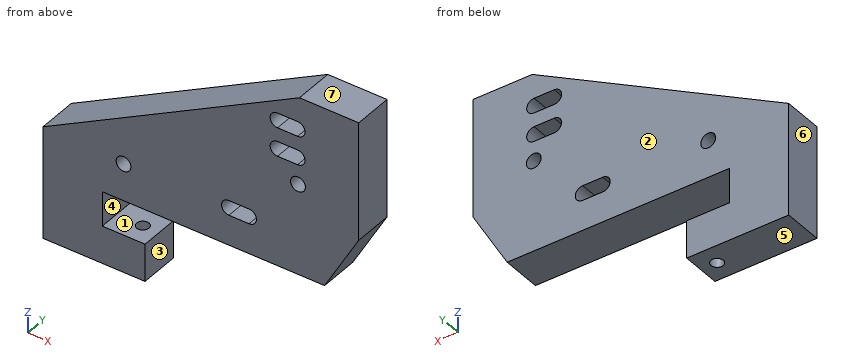
from build123d import *

# Parameters (mm, degrees)
F1_DEPTH = 25.4
F2_R     = 4.7625
F3_DEPTH = 25.401
F5_D     = 7.9375
F5_DEPTH = 25.4
F5_TIP   = 2.3846655818


with BuildPart() as f1:
    # F0 (on Front) → F1 (new body)
    with BuildSketch(Plane.XZ):
        Polygon((0, 72.3138), (0, 0), (65.5828, 0), (65.5828, 24.1554), (38.1, 24.1554), (38.1, 46.4693), (180.975, 46.4693), (202.9293194803, 85.1191428995), (202.9293194803, 161.3191428995), (164.8293194803, 161.3191428995), align=None)
    extrude(amount=F1_DEPTH)

    # F2 (on face) → F3 (cut, through all)
    with BuildSketch(Plane.XZ.offset(25.4)):
        with Locations((51.7525, 70.2818)):
            Circle(F2_R)
        with Locations((163.8768194803, 104.8766)):
            Circle(F2_R)
        with BuildLine():
            Line((132.3975, 75.3999), (119.4943, 75.3999))
            ThreePointArc((119.4943, 75.3999), (114.7318, 70.6374), (119.4943, 65.8749))
            Line((119.4943, 65.8749), (132.3975, 65.8749))
            ThreePointArc((132.3975, 65.8749), (137.16, 70.6374), (132.3975, 75.3999))
        make_face()
        with BuildLine():
            Line((163.6482194803, 145.3769), (150.7450194803, 145.3769))
            ThreePointArc((150.7450194803, 145.3769), (145.9825194803, 140.6144), (150.7450194803, 135.8519))
            Line((150.7450194803, 135.8519), (163.6482194803, 135.8519))
            ThreePointArc((163.6482194803, 135.8519), (168.4107194803, 140.6144), (163.6482194803, 145.3769))
        make_face()
        with BuildLine():
            Line((163.6482194803, 126.9619), (150.7450194803, 126.9619))
            ThreePointArc((150.7450194803, 126.9619), (145.9825194803, 122.1994), (150.7450194803, 117.4369))
            Line((150.7450194803, 117.4369), (163.6482194803, 117.4369))
            ThreePointArc((163.6482194803, 117.4369), (168.4107194803, 122.1994), (163.6482194803, 126.9619))
        make_face()
    extrude(amount=-F3_DEPTH, mode=Mode.SUBTRACT)

    # F5
    with Locations(Plane(origin=(0, 0, 0), x_dir=(1, 0, 0), z_dir=(0, 0, -1))):
        with Locations((55.0799, 12.7)):
            Hole(F5_D / 2, depth=F5_DEPTH)
            with Locations((0, 0, -(F5_DEPTH + F5_TIP / 2))):  # 118° drill point
                Cone(0, F5_D / 2, F5_TIP, mode=Mode.SUBTRACT)


solid = f1.part
Could you check a few things on this model? Use its own coordinates, in mm. Face numbers are marked on the shaded views. A direction names the side the tool comes from. Round coordinates to 2 decimals unless told otherwise and drop trailing zeros. Write each loop counter-clockwise with the first axis right and the second up, starting at its lowest first coordinate (ties: lowest second). Pieces come first, ordered by that corner, then holes. Notation, with made-up numbers: (-29, -33) - (-2, -33) arc R23 ccw to (-2, -21) - close; hole circle Ø11 at (67, 74.25). An arc over 180 degrees is marked (long way). Use a Markdown table: item, result.
Q1. For pin 1 (14 mm diameter, centred on x = 126, y = -17, fed in from -Z); pin 2 (4 mm diameter, centred on x = 126.5, y = -17, fed in from +Z); pin 3 (3 mm diameter, centred on y = -21, z = 75, fed in from -X); pin 4 (7.5 mm diameter, centred on x = 163.88, z = 104.88, fed in from +Y), each with a flat end and sliding along its axis, tell me the tip position at first contact or that it passes through.
Output values:
| item | result |
|---|---|
| pin 1 | z = 46.47 |
| pin 2 | z = 141.7 |
| pin 3 | x = 2.2 |
| pin 4 | through |
Q2. I want a section at C-C (z = 38). List the corners of the cut face in (x, y) for me, plus the area to 3 significant figures.
Output values:
| item | result |
|---|---|
| outline | (0, -25.4) - (38.1, -25.4) - (38.1, 0) - (0, 0) - close |
| area | 968 mm2 |
Q3. I want a section at B-B (y = -22). List the corners of the cut face in (x, z) for me (1 decimal), plus the area to 3 significant figures.
Output values:
| item | result |
|---|---|
| outline | (0, 0) - (65.6, 0) - (65.6, 24.2) - (38.1, 24.2) - (38.1, 46.5) - (181, 46.5) - (202.9, 85.1) - (202.9, 161.3) - (164.8, 161.3) - (0, 72.3) - close; hole circle Ø9.5 at (51.8, 70.3); hole (119.5, 65.9) - (132.4, 65.9) arc R4.8 ccw to (132.4, 75.4) - (119.5, 75.4) arc R4.8 ccw to start; hole (150.7, 117.4) - (163.6, 117.4) arc R4.8 ccw to (163.6, 127) - (150.7, 127) arc R4.8 ccw to start; hole (150.7, 135.9) - (163.6, 135.9) arc R4.8 ccw to (163.6, 145.4) - (150.7, 145.4) arc R4.8 ccw to start; hole circle Ø9.5 at (163.9, 104.9) |
| area | 17,300 mm2 |
Q4. I want a section at D-D (x = 189). List the corners of the cut face in (y, z) for me, plus the area to 3 significant figures.
Output values:
| item | result |
|---|---|
| outline | (-25.4, 60.6) - (0, 60.6) - (0, 161.32) - (-25.4, 161.32) - close |
| area | 2,560 mm2 |
Q5. I want a section at A-A (y = -12.7). List the corners of the cut face in (x, z) for me (1 decimal), plus the area to 3 significant figures.
Output values:
| item | result |
|---|---|
| outline | (0, 0) - (51.1, 0) - (51.1, 24.2) - (38.1, 24.2) - (38.1, 46.5) - (181, 46.5) - (202.9, 85.1) - (202.9, 161.3) - (164.8, 161.3) - (0, 72.3) - close; (59, 0) - (65.6, 0) - (65.6, 24.2) - (59, 24.2) - close; hole circle Ø9.5 at (51.8, 70.3); hole (119.5, 65.9) - (132.4, 65.9) arc R4.8 ccw to (132.4, 75.4) - (119.5, 75.4) arc R4.8 ccw to start; hole (150.7, 117.4) - (163.6, 117.4) arc R4.8 ccw to (163.6, 127) - (150.7, 127) arc R4.8 ccw to start; hole (150.7, 135.9) - (163.6, 135.9) arc R4.8 ccw to (163.6, 145.4) - (150.7, 145.4) arc R4.8 ccw to start; hole circle Ø9.5 at (163.9, 104.9) |
| area | 17,100 mm2 |
Q6. Please list where these lines run through material, in increasing order: L1, parallel to Z at x = 149.5, y = -21.25; L2, parallel to Z at x = 167, y = -4; L3, parallel to X at y = -9.5, z = 103.
Output values:
| item | result |
|---|---|
| L1 | 46.47 to 117.6, 126.8 to 136.02, 145.21 to 153.04 |
| L2 | 46.47 to 101.28, 108.47 to 118.82, 125.58 to 137.23, 144 to 161.32 |
| L3 | 56.83 to 159.5, 168.25 to 202.93 |
Q7. Thinking about a two-plate mould opening in Z: for the marked faces 4, 5, 6 and 7, which applies, released by +Z, released by -Z, zero draft, split by the parting line, or undercut?
Output values:
| item | result |
|---|---|
| face 4 | undercut |
| face 5 | released by -Z |
| face 6 | zero draft |
| face 7 | released by +Z |
Q8. For the marked faces 1, 2 and 3, which set-ups out of +Z, -Z, +X, -X, +Y, -Y let a thin tool reach every point of the face, with its end or its side?
Output values:
| item | result |
|---|---|
| face 1 | +X, +Y, -Y |
| face 2 | +Z, -Z, +X, -X, +Y |
| face 3 | -Z, +X, +Y, -Y |
